from build123d import *

# Parameters (mm, degrees)
BOSS_EXTRUDE1_DEPTH          = 11
SKETCH2_R                    = 6.53025
BOSS_EXTRUDE2_DEPTH          = 16.000051
F_6_0_6_DIAMETER_HOLE1_D     = 6
F_6_0_6_DIAMETER_HOLE1_DEPTH = 22.000051
SKETCH6_R                    = 0.016569
CUT_EXTRUDE1_DEPTH           = 80
SKETCH7_R                    = 3
CUT_EXTRUDE2_DEPTH           = 80
SKETCH8_R                    = 1.5
CUT_EXTRUDE3_DEPTH           = 11.336659
CUT_EXTRUDE3_DEPTH_BACK      = 9.444233


with BuildPart() as part:
    # Sketch1 → Boss-Extrude1 (new body)
    with BuildSketch(Plane(origin=(10.625148, 0, 0), x_dir=(0, 0, -1), z_dir=(1, 0, 0))):
        with BuildLine():
            ThreePointArc((-3.411257, 6.887327), (-4.211338, 6.495564), (-4.950655, 5.998555))
            ThreePointArc((-4.950655, 5.998555), (-5.965428, 7.279572), (-7.470402, 7.916612))
            ThreePointArc((-7.470402, 7.916612), (-7.752116, 7.646104), (-8.022623, 7.364391))
            ThreePointArc((-8.022623, 7.364391), (-7.385583, 5.859416), (-6.104566, 4.844644))
            ThreePointArc((-6.104566, 4.844644), (-6.601575, 4.105327), (-6.993338, 3.305246))
            ThreePointArc((-6.993338, 3.305246), (-8.512666, 3.907253), (-10.134532, 3.706458))
            ThreePointArc((-10.134532, 3.706458), (-10.243249, 3.331335), (-10.336659, 2.95211))
            ThreePointArc((-10.336659, 2.95211), (-9.032479, 1.967284), (-7.415699, 1.728974))
            ThreePointArc((-7.415699, 1.728974), (-7.476463, 0.840202), (-7.415699, -0.04857))
            ThreePointArc((-7.415699, -0.04857), (-9.032479, -0.28688), (-10.336659, -1.271707))
            ThreePointArc((-10.336659, -1.271707), (-10.243249, -1.650932), (-10.134532, -2.026055))
            ThreePointArc((-10.134532, -2.026055), (-8.512666, -2.226849), (-6.993338, -1.624842))
            ThreePointArc((-6.993338, -1.624842), (-6.601575, -2.424923), (-6.104566, -3.16424))
            ThreePointArc((-6.104566, -3.16424), (-7.385583, -4.179013), (-8.022623, -5.683988))
            ThreePointArc((-8.022623, -5.683988), (-7.752116, -5.965701), (-7.470402, -6.236208))
            ThreePointArc((-7.470402, -6.236208), (-5.965428, -5.599169), (-4.950655, -4.318152))
            ThreePointArc((-4.950655, -4.318152), (-4.211338, -4.815161), (-3.411257, -5.206923))
            ThreePointArc((-3.411257, -5.206923), (-4.013264, -6.726251), (-3.812469, -8.348117))
            ThreePointArc((-3.812469, -8.348117), (-3.437346, -8.456834), (-3.058122, -8.550244))
            ThreePointArc((-3.058122, -8.550244), (-2.073295, -7.246064), (-1.834985, -5.629284))
            ThreePointArc((-1.834985, -5.629284), (-0.946213, -5.690048), (-0.057441, -5.629284))
            ThreePointArc((-0.057441, -5.629284), (0.180869, -7.246064), (1.165696, -8.550244))
            ThreePointArc((1.165696, -8.550244), (1.54492, -8.456834), (1.920043, -8.348117))
            ThreePointArc((1.920043, -8.348117), (2.120838, -6.726251), (1.518831, -5.206923))
            ThreePointArc((1.518831, -5.206923), (2.318912, -4.815161), (3.058229, -4.318152))
            ThreePointArc((3.058229, -4.318152), (4.073002, -5.599169), (5.577976, -6.236208))
            ThreePointArc((5.577976, -6.236208), (5.85969, -5.965701), (6.130197, -5.683988))
            ThreePointArc((6.130197, -5.683988), (5.493157, -4.179013), (4.21214, -3.16424))
            ThreePointArc((4.21214, -3.16424), (4.709149, -2.424923), (5.100912, -1.624842))
            ThreePointArc((5.100912, -1.624842), (6.62024, -2.226849), (8.242106, -2.026055))
            ThreePointArc((8.242106, -2.026055), (8.350823, -1.650932), (8.444233, -1.271707))
            ThreePointArc((8.444233, -1.271707), (7.140053, -0.28688), (5.523273, -0.04857))
            ThreePointArc((5.523273, -0.04857), (5.584037, 0.840202), (5.523273, 1.728974))
            ThreePointArc((5.523273, 1.728974), (7.140053, 1.967284), (8.444233, 2.95211))
            ThreePointArc((8.444233, 2.95211), (8.350823, 3.331335), (8.242106, 3.706458))
            ThreePointArc((8.242106, 3.706458), (6.62024, 3.907253), (5.100912, 3.305246))
            ThreePointArc((5.100912, 3.305246), (4.709149, 4.105327), (4.21214, 4.844644))
            ThreePointArc((4.21214, 4.844644), (5.493157, 5.859416), (6.130197, 7.364391))
            ThreePointArc((6.130197, 7.364391), (5.85969, 7.646104), (5.577976, 7.916612))
            ThreePointArc((5.577976, 7.916612), (4.073002, 7.279572), (3.058229, 5.998555))
            ThreePointArc((3.058229, 5.998555), (2.318912, 6.495564), (1.518831, 6.887327))
            ThreePointArc((1.518831, 6.887327), (2.120838, 8.406654), (1.920043, 10.02852))
            ThreePointArc((1.920043, 10.02852), (1.54492, 10.137238), (1.165696, 10.230647))
            ThreePointArc((1.165696, 10.230647), (0.180869, 8.926467), (-0.057441, 7.309688))
            ThreePointArc((-0.057441, 7.309688), (-0.946213, 7.370452), (-1.834985, 7.309688))
            ThreePointArc((-1.834985, 7.309688), (-2.073295, 8.926467), (-3.058122, 10.230647))
            ThreePointArc((-3.058122, 10.230647), (-3.437346, 10.137238), (-3.812469, 10.02852))
            ThreePointArc((-3.812469, 10.02852), (-4.013264, 8.406654), (-3.411257, 6.887327))
        make_face()
    extrude(amount=-BOSS_EXTRUDE1_DEPTH)

    # Sketch2 → Boss-Extrude2 (add)
    with BuildSketch(Plane.ZY.offset(0.374852)):
        with Locations((0.946213, 0.840202)):
            Circle(SKETCH2_R)
    extrude(amount=BOSS_EXTRUDE2_DEPTH)

    # Ø6.0 (6) Diameter Hole1
    with Locations(Plane(origin=(10.625148, 0, 0), x_dir=(0, 0, -1), z_dir=(1, 0, 0))):
        with Locations((-0.946213, 0.840202)):
            Hole(F_6_0_6_DIAMETER_HOLE1_D / 2, depth=F_6_0_6_DIAMETER_HOLE1_DEPTH)

    # Sketch6 → Cut-Extrude1 (cut)
    with BuildSketch(Plane(origin=(10.625148, 0, 0), x_dir=(0, 0, -1), z_dir=(1, 0, 0))):
        with Locations((-0.399147, -2.092643)):
            Circle(SKETCH6_R)
    extrude(amount=-CUT_EXTRUDE1_DEPTH, mode=Mode.SUBTRACT)

    # Sketch7 → Cut-Extrude2 (cut)
    with BuildSketch(Plane(origin=(10.625148, 0, 0), x_dir=(0, 0, -1), z_dir=(1, 0, 0))):
        with Locations((-0.946213, 0.840202)):
            Circle(SKETCH7_R)
    extrude(amount=-CUT_EXTRUDE2_DEPTH, mode=Mode.SUBTRACT)

    # Sketch8 → Cut-Extrude3 (cut, two sides)
    with BuildSketch(Plane.XY) as cut_extrude3_sk:
        with Locations((-9.449872, 0)):
            Circle(SKETCH8_R)
    extrude(amount=CUT_EXTRUDE3_DEPTH, mode=Mode.SUBTRACT)
    extrude(cut_extrude3_sk.sketch, amount=-CUT_EXTRUDE3_DEPTH_BACK, mode=Mode.SUBTRACT)


solid = part.part
Model file for the job. Use its own axes, mm. Give positions to 0.01 mm unless a question says otherwise; leave off trailing zeros. Order: outer loops, then holes, each group sorted by start corner. A loop starts at its lowest first (then second) coordinate and runs counter-clockwise, first axis right, second up. Notation, with made-up numbers: (20, 82) - (33, 82) arc R19 ccw to (33, 106) - close; hole circle Ø8 at (38, 72). An arc over 180 degrees is marked (long way). Write item = value, one per line. Start each with the question number.
1. Cut at B-B, the plane x = -6.5. List the corners of the cut face in (y, z).
2. Drop flat-ended pins along their axis: P1, Ø1.1, axis at y = 8, z = -1.5, coming from the -X side; P2, Ø4, axis at x = -13, y = -4, coming from the +Z side; P3, Ø1.8, axis at x = -9.45, y = 0, coming from the -Z side; P4, Ø2, axis at x = -4.5, z = 5.5, coming from the -Y side. Give the stop position or say it passes through.
3. Probe line 1 along X through (y, z) = (0, -4.45); line 2 along Y through (x, z) = (4, 1); line 3 along X through (y, z) = (6, -4.75). List the from-to ranges inside material, lowest first.
4. Two-plate mould, pull along X, no slides. Class faces 1 (the flat face through (-0.375, 6, 7)), 2 (the cylindrical face through (-9.775, -1.464, -3.742)): pulls with the +X half, pulls with the -X half, needs draft (parallel to the pull), parting line crosses it, or undercut.
Taken from the geometry:
q1.outline = circle Ø13.06 at (0.84, 0.95); hole circle Ø6 at (0.84, 0.95)
q2.P1 = -0.37
q2.P2 = 6.83
q2.P3 = through
q2.P4 = -4.64
q3.line_1 = -16.37 to -10.95, -7.95 to 10.63
q3.line_2 = -5.69 to -2.16, 3.84 to 7.37
q3.line_3 = -0.37 to 10.63
q4.face_1 = pulls with the -X half
q4.face_2 = undercut
